The model under review builds one solid part; all positions refer to its coordinate system, in mm. A direction names the side the tool comes from. Round coordinates to 2 decimals unless told otherwise and drop trailing zeros. Order: outer loops, then holes, each group sorted by start corner. A loop starts at its lowest first (then second) coordinate and runs counter-clockwise, first axis right, second up. Notation, with made-up numbers: (82.5, 22) -> (98.5, 22) arc R29 ccw to (98.5, 50) -> close; hole circle Ø6 at (47.25, 80.5). An arc over 180 degrees is marked (long way). Put each result on its own line as item: value. Start each with the question number.
from build123d import *

# Parameters (mm, degrees)
PAD_DEPTH    = 4.5
CHAMFER_SIZE = 0.35


with BuildPart() as part:
    # Sketch → Revolution (revolve)
    with BuildSketch(Plane(origin=(0, 0, 0), x_dir=(-1, 0, 0), z_dir=(0, 1, 0))):
        with BuildLine():
            Line((0, 0), (1.163333, 0))
            ThreePointArc((1.163333, 0), (1.224616, 0.025384), (1.25, 0.086667))
            Line((1.25, 0.086667), (1.25, 0.413333))
            ThreePointArc((1.25, 0.413333), (1.224616, 0.474616), (1.163333, 0.5))
            Line((1.163333, 0.5), (0.65, 0.5))
            Line((0.65, 0.5), (0.65, 6.3375))
            ThreePointArc((0.65, 6.3375), (0.602405, 6.452405), (0.4875, 6.5))
            Line((0.4875, 6.5), (0, 6.5))
            Line((0, 6.5), (0, 0))
        make_face()
    revolve(axis=Axis((0, 0, 0), (0, 0, 1)))

    # Sketch001 → Pad (new body)
    with BuildSketch(Plane.XY):
        Polygon((-0.7, 0), (0, 0.7), (0.7, 0), (0, -0.7), align=None)
    extrude(amount=-PAD_DEPTH)

    # Chamfer
    chamfer_edges = [part.edges().sort_by_distance(p)[0] for p in [
        (0.35, -0.35, -4.5),
        (-0.35, -0.35, -4.5),
        (-0.35, 0.35, -4.5),
        (0.35, 0.35, -4.5),
    ]]
    chamfer(chamfer_edges, length=CHAMFER_SIZE)


solid = part.part
Q1. Wall thickness on probe 1 along X at (y, z) = (0.05, 3.5); probe 2 along Z at (x, y) = (0, 1.1); probe 3 along Y at (x, z) = (-0.2, -2.25): over which ranges is each line inside the solid? List them lowest first. Write a range as [from, to].
Q2. Clearance check with flat-ended pins moving along their axes: pin 1 Ø1.5 at (x, z) = (1, 5) entering from +Y; pin 2 Ø1.5 at (x, z) = (0.5, -2) entering from +Y. State where each tip first meets the part, or that it passes through.
Q3. Take a section at A-A on z = 4.75. Give the boundary of the cut face in (x, y), and give its area (3 significant figures).
Q4. For faces 1 (the face through (0.085, -0.644, 3.46)), 2 (the face through (0, 0, 6.5)), 3 (the face through (0, 1, 0)), list the 3-axis set-ups (+Z, -Z, +X, -X, +Y, -Y) from which the entire face can be reached by the end or side of a thin tool; tool diameter is ignored.
Calculated:
1. probe 1: x = [-0.65, 0.65]
1. probe 2: z = [0, 0.5]
1. probe 3: y = [-0.5, 0.5]
2. pin 1: stops at y = 0.6
2. pin 2: stops at y = 0.7
3. outline: circle Ø1.3 at (0, 0)
3. area: 1.33 mm²
4. face 1: +Z
4. face 2: +Z, +X, -X, +Y, -Y
4. face 3: -Z
